Read the model definition and answer for the solid it produces. Units are mm, in the model's axes. A direction names the side the tool comes from. Round coordinates to 2 decimals unless told otherwise and drop trailing zeros. Order: outer loops, then holes, each group sorted by start corner. A loop starts at its lowest first (then second) coordinate and runs counter-clockwise, first axis right, second up. Notation, with made-up numbers: (35.5, 30) - (85.5, 30) arc R24 cw to (85.5, 65) - close; hole circle Ø2 at (-12.75, 77). An arc over 180 degrees is marked (long way). Put each result on its own line as item: value. Start each with the question number.
Q1. Section A-A on x = 0 is taken. Give the vertices of the cut face in (y, z), then the cut area to 3 significant figures.
Q2. Section C-C on z = 30.5 is taken. Give the vertices of the cut face in (x, y).
Q3. Which of the six approach directions +Z, -Z, +X, -X, +Y, -Y give full straight-line access (tool end or side, diameter ignored) to faces 1 (the face through (-6, 8.173, 27)), 2 (the face through (-6, -8.173, 27)), 3 (the face through (24.627, 0, 42)), 4 (the face through (-18.56, 0.17, 59.13)), 5 (the face through (12.313, 0, 47))?
Q4. Section B-B on y = 0 is taken. Give the vertices of the cut face in (x, z).
Q5. Find the intervals of material crossed by line 1 along X through (y, z) = (0, 6); line 2 along Z through (x, y) = (-17.25, 0); line 3 along Z through (x, y) = (-23.5, -9), in increasing order. Write a range as from..to.
Q6. Each of these flat-tipped pins is pushed along its axis until it touches: pin 1 Ø11 at (y, z) = (0, 50.95) entering from +X; pin 2 Ø12 at (x, y) = (-17.5, -6.5) entering from +Z; pin 3 Ø3 at (y, z) = (5.5, 8.5) entering from +X. Where does it stop, or does it pass through?
Q7. Section D-D on y = -5.5 is taken. Give the vertices of the cut face in (x, z).
Q8. For a pull along X with two mould halves and no side action, classify faces 6 (the face through (-24.627, 0, 42)), 7 (the face through (-18.556, 0.444, 54.332)), 8 (the face through (-0.27, -0.11, 26.55)) as pulls with the +X half, pulls with the -X half, needs draft (parallel to the pull), parting line crosses it, or undercut.
from build123d import *

# Parameters (mm, degrees)
F0_W     = 49.2534674704
F0_H     = 16.3461286575
F1_DEPTH = 25.4
F2_DEPTH = 43.942
F4_DEPTH = 25.4
F5_DEPTH = 16.51
F7_DEPTH = 78.486
F8_R     = 3.4125622967
F9_DEPTH = 57.15


with BuildPart() as f1:
    # F0 (on Top) → F1 (new body)
    with BuildSketch(Plane.XY):
        with BuildLine():
            Line((45.9197200835, 7.0321863355), (45.9197200835, 17.6366120577))
            Line((45.9197200835, 17.6366120577), (-45.9197200835, 17.6366120577))
            Line((-45.9197200835, 17.6366120577), (-45.9197200835, 7.0321863355))
            ThreePointArc((-45.9197200835, 7.0321863355), (-40.9472134391, 4.9725066444), (-38.887533748, 0))
            ThreePointArc((-38.887533748, 0), (-40.9472134391, -4.9725066444), (-45.9197200835, -7.0321863355))
            Line((-45.9197200835, -7.0321863355), (-45.9197200835, -17.6366120577))
            Line((-45.9197200835, -17.6366120577), (45.9197200835, -17.6366120577))
            Line((45.9197200835, -17.6366120577), (45.9197200835, -7.0321863355))
            ThreePointArc((45.9197200835, -7.0321863355), (38.887533748, 0), (45.9197200835, 7.0321863355))
        make_face()
        Rectangle(F0_W, F0_H, mode=Mode.SUBTRACT)
        with BuildLine():
            ThreePointArc((45.9197200835, -17.6366120577), (63.5563321412, 0), (45.9197200835, 17.6366120577))
            Line((45.9197200835, 17.6366120577), (45.9197200835, 7.0321863355))
            ThreePointArc((45.9197200835, 7.0321863355), (50.8922267279, 4.9725066444), (52.951906419, 0))
            ThreePointArc((52.951906419, 0), (50.8922267279, -4.9725066444), (45.9197200835, -7.0321863355))
            Line((45.9197200835, -7.0321863355), (45.9197200835, -17.6366120577))
        make_face()
        with BuildLine():
            Line((-45.9197200835, 7.0321863355), (-45.9197200835, 17.6366120577))
            ThreePointArc((-45.9197200835, 17.6366120577), (-63.5563321412, 0), (-45.9197200835, -17.6366120577))
            Line((-45.9197200835, -17.6366120577), (-45.9197200835, -7.0321863355))
            ThreePointArc((-45.9197200835, -7.0321863355), (-52.951906419, 0), (-45.9197200835, 7.0321863355))
        make_face()
    extrude(amount=F1_DEPTH)

    # F0 (on Top) → F2 (join)
    with BuildSketch(Plane.XY):
        Rectangle(F0_W, F0_H)
    extrude(amount=F2_DEPTH)

    # F3 (on face) → F4 (cut)
    with BuildSketch(Plane.XZ.offset(8.1730643287)):
        with BuildLine():
            Line((0, 43.942), (-12.3133668676, 43.942))
            Line((-12.3133668676, 43.942), (-12.3133668676, 38.862))
            ThreePointArc((-12.3133668676, 38.862), (0, 26.5486331324), (12.3133668676, 38.862))
            Line((12.3133668676, 38.862), (12.3133668676, 43.942))
            Line((12.3133668676, 43.942), (0, 43.942))
        make_face()
    extrude(amount=-F4_DEPTH, mode=Mode.SUBTRACT)

    # F5 (add): faces of the model
    f5_faces = [f1.faces().sort_by_distance(p)[0] for p in [
        (-18.4700503014, 0, 43.942),
        (18.4700503014, 0, 43.942),
    ]]
    extrude(f5_faces, amount=F5_DEPTH)

    # F6 (on face) → F7 (cut)
    with BuildSketch(Plane(origin=(-24.6267337352, 0, 0), x_dir=(0, -1, 0), z_dir=(-1, 0, 0))):
        with BuildLine():
            ThreePointArc((-8.1730643287, 51.3854473829), (0, 59.1332048708), (8.1730643287, 51.3854473829))
            Line((8.1730643287, 51.3854473829), (8.1730643287, 60.452))
            Line((8.1730643287, 60.452), (-8.1730643287, 60.452))
            Line((-8.1730643287, 60.452), (-8.1730643287, 51.3854473829))
        make_face()
    extrude(amount=-F7_DEPTH, mode=Mode.SUBTRACT)

    # F8 (on face) → F9 (cut)
    with BuildSketch(Plane(origin=(-24.6267337352, 0, 0), x_dir=(0, -1, 0), z_dir=(-1, 0, 0))):
        with Locations((0, 50.9484671056)):
            Circle(F8_R)
    extrude(amount=-F9_DEPTH, mode=Mode.SUBTRACT)


solid = f1.part
Findings:
1. outline: (-17.64, 0) - (17.64, 0) - (17.64, 25.4) - (8.17, 25.4) - (8.17, 26.55) - (-8.17, 26.55) - (-8.17, 25.4) - (-17.64, 25.4) - close
1. area: 915 mm2
2. outline: (-24.63, -8.17) - (-9.04, -8.17) - (-9.04, 8.17) - (-24.63, 8.17) - close; (9.04, -8.17) - (24.63, -8.17) - (24.63, 8.17) - (9.04, 8.17) - close
3. face 1: +Z, +X, -X, +Y
3. face 2: +Z, +X, -X, -Y
3. face 3: +Z, +X, +Y, -Y
3. face 4: +Z, +X, -X
3. face 5: +Z, +Y, -Y
4. outline: (-63.56, 0) - (-52.95, 0) - (-52.95, 25.4) - (-63.56, 25.4) - close; (-38.89, 0) - (38.89, 0) - (38.89, 25.4) - (24.63, 25.4) - (24.63, 47.54) - (12.31, 47.54) - (12.31, 38.86) arc R12.31 cw to (-12.31, 38.86) - (-12.31, 47.54) - (-24.63, 47.54) - (-24.63, 25.4) - (-38.89, 25.4) - close; (-24.63, 54.36) - (-12.31, 54.36) - (-12.31, 59.13) - (-24.63, 59.13) - close; (12.31, 54.36) - (24.63, 54.36) - (24.63, 59.13) - (12.31, 59.13) - close; (52.95, 0) - (63.56, 0) - (63.56, 25.4) - (52.95, 25.4) - close
5. line 1: -63.56..-52.95, -38.89..38.89, 52.95..63.56
5. line 2: 0..47.54, 54.36..59.13
5. line 3: 0..25.4
6. pin 1: x = 24.63
6. pin 2: z = 59.12
6. pin 3: x = 63.1
7. outline: (-62.68, 0) - (-50.3, 0) - (-50.3, 25.4) - (-62.68, 25.4) - close; (-41.54, 0) - (41.54, 0) - (41.54, 25.4) - (24.63, 25.4) - (24.63, 57.01) - (12.31, 57.01) - (12.31, 38.86) arc R12.31 cw to (-12.31, 38.86) - (-12.31, 57.01) - (-24.63, 57.01) - (-24.63, 25.4) - (-41.54, 25.4) - close; (50.3, 0) - (62.68, 0) - (62.68, 25.4) - (50.3, 25.4) - close
8. face 6: pulls with the -X half
8. face 7: needs draft
8. face 8: undercut
